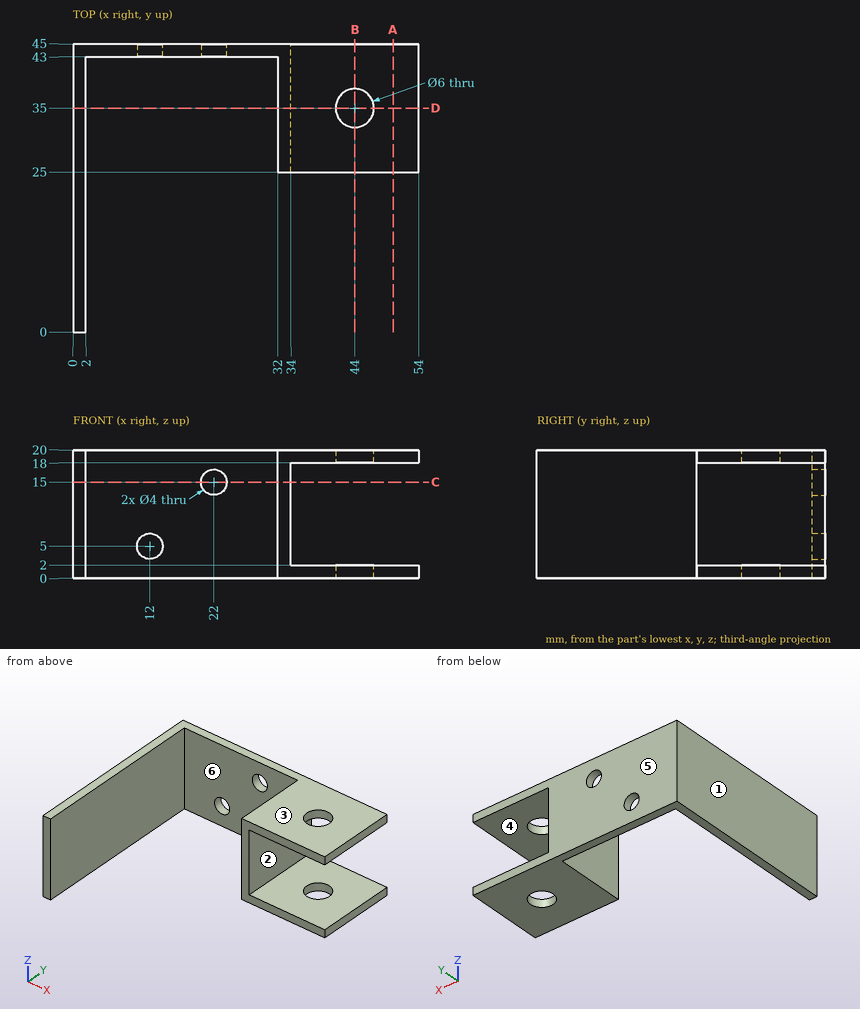
Print and shaded views of the part. All mm, measured from the part's lowest x, y and z. A direction names the side the tool comes from. Round coordinates to 2 decimals unless told otherwise and drop trailing zeros. Write each loop counter-clockwise with the first axis right and the second up, starting at its lowest first coordinate (ties: lowest second). Pieces come first, ordered by that corner, then holes. Notation, with made-up numbers: M 8,25 L 28,25 A7 ccw 28,32 Z; hole C 17.5,62.5 d2. An arc over 180 degrees is marked long. One line per question, with ' | ' between items.
(1) Probe line 1 along X through (y, z) = (35, 0.75); line 2 along X through (y, z) = (30, 17.25); line 3 along Y through (x, z) = (44, 19.35). List the from-to ranges inside material, lowest first.
Answer key:
line 1: x = 0 to 2, 32 to 41, 47 to 54 | line 2: x = 0 to 2, 32 to 34 | line 3: y = 25 to 32, 38 to 45
(2) Saw through at C-C on z = 15. Write the cut outline in (x, y), then the cut area to 3 significant figures.
Answer key:
outline: M 0,0 L 2,0 L 2,43 L 20,43 L 20,45 L 0,45 Z; M 24,43 L 32,43 L 32,25 L 34,25 L 34,45 L 24,45 Z | area: 182 mm^2
(3) Pin check, flat tips, straight feed: pin 1 (10 mm diameter, centred on x = 21, z = 8, fed in from -Y); pin 2 (8 mm diameter, centred on y = 9.5, z = 10, fed in from +X). Stop position of each tip, or through.
Answer key:
pin 1: stops at y = 43 | pin 2: stops at x = 2
(4) Two-plate mould, pull along Z, no slides. Class the marked faces 1, 2 and 3: released by +Z, released by -Z, zero draft, split by the parting line, or undercut.
Answer key:
face 1: zero draft | face 2: undercut | face 3: released by +Z
(5) Saw through at A-A on x = 50. Write the cut outline in (y, z).
Answer key:
outline: M 25,0 L 45,0 L 45,2 L 25,2 Z; M 25,18 L 45,18 L 45,20 L 25,20 Z
(6) Saw through at B-B on x = 44. Write the cut outline in (y, z), then the cut area to 3 significant figures.
Answer key:
outline: M 25,0 L 32,0 L 32,2 L 25,2 Z; M 25,18 L 32,18 L 32,20 L 25,20 Z; M 38,0 L 45,0 L 45,2 L 38,2 Z; M 38,18 L 45,18 L 45,20 L 38,20 Z | area: 56.0 mm^2
(7) 3-axis set-ups, long thin cutter, end or side, ignore diameter. For the marked faces 4, 5 and 6: which of +Z, -Z, +X, -X, +Y, -Y reach the whole face in a straight line?
Answer key:
face 4: +X, +Y, -Y | face 5: +Z, -Z, +X, -X, +Y | face 6: +Z, -Z, -Y
(8) Saw through at D-D on y = 35. Write the cut outline in (x, z).
Answer key:
outline: M 0,0 L 2,0 L 2,20 L 0,20 Z; M 32,0 L 41,0 L 41,2 L 34,2 L 34,18 L 41,18 L 41,20 L 32,20 Z; M 47,0 L 54,0 L 54,2 L 47,2 Z; M 47,18 L 54,18 L 54,20 L 47,20 Z
